Design review of the part built by this model. Coordinates are the model's own, in mm. Face numbers are marked on the shaded views. A direction names the side the tool comes from. Give positions to 0.01 mm unless a question says otherwise; leave off trailing zeros. Write each loop counter-clockwise with the first axis right and the second up, starting at its lowest first coordinate (ties: lowest second). Pieces come first, ordered by that corner, then holes.
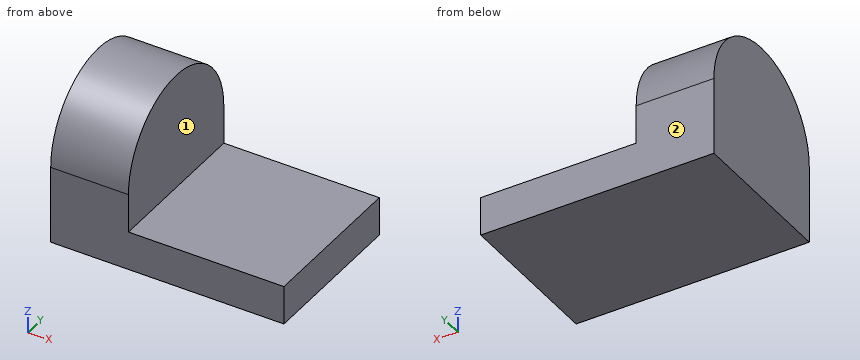
```python
from build123d import *

# Parameters (mm, degrees)
F0_W     = 152.4
F0_H     = 101.6
F1_DEPTH = 25.4
F2_W     = 101.6
F2_H     = 25.4
F3_DEPTH = 50.8


with BuildPart() as f1:
    # F0 (on Top) → F1 (new body)
    with BuildSketch(Plane.XY):
        with Locations((-76.2, 50.8)):
            Rectangle(F0_W, F0_H)
    extrude(amount=F1_DEPTH)

    # F2 (on face) → F3 (join)
    with BuildSketch(Plane(origin=(-152.4, 0, 0), x_dir=(0, -1, 0), z_dir=(-1, 0, 0))):
        with Locations((-50.8, 38.1)):
            Rectangle(F2_W, F2_H)
        with BuildLine():
            ThreePointArc((0, 50.8), (-50.8, 101.6), (-101.6, 50.8))
            Line((-101.6, 50.8), (0, 50.8))
        make_face()
    extrude(amount=-F3_DEPTH)


solid = f1.part
```
(1) Consider section C-C, the plane z = 36. Give the boundary of the cut face in (x, y).
Resolved:
outline: (-152.4, 0) - (-101.6, 0) - (-101.6, 101.6) - (-152.4, 101.6) - close
(2) To check wall thickness, follow L1, parallel to X at y = 15, z = 75.5; L2, parallel to Z at x = -117, y = 49.5; L3, parallel to Z at x = -33, y = 90. State the ranges of each line that lie inside material, in increasing order.
Resolved:
L1: x = -152.4 to -101.6
L2: z = 0 to 101.58
L3: z = 0 to 25.4
(3) Consider section A-A, the plane y = 50.8. Give the boundary of the cut face in (x, z).
Resolved:
outline: (-152.4, 0) - (0, 0) - (0, 25.4) - (-101.6, 25.4) - (-101.6, 101.6) - (-152.4, 101.6) - close
(4) Tool access review of the marked faces 1 and 2: name each direction out of +Z, -Z, +X, -X, +Y, -Y from which nothing blocks a thin tool from reaching the whole face with its end or side.
Resolved:
face 1: +Z, +X, +Y, -Y
face 2: +Z, -Z, +X, -X, +Y
(5) Clearance check with flat-ended pins moving along their axes: P1, Ø12, axis at x = -27.5, y = 20, coming from the +Z side; P2, Ø4, axis at x = -98.5, z = 54.5, coming from the +Y side (3 decimals); P3, Ø5, axis at y = 16.5, z = 62.5, coming from the +X side. State where each tip first meets the part, or that it passes through.
Resolved:
P1: stops at z = 25.4
P2: passes through
P3: stops at x = -101.6
(6) Consider section B-B, the plane x = -21. Give the boundary of the cut face in (y, z), then the cut area to 3 significant figures.
Resolved:
outline: (0, 0) - (101.6, 0) - (101.6, 25.4) - (0, 25.4) - close
area: 2,580 mm2
(7) Consider section D-D, the plane y = 82. Give the boundary of the cut face in (x, z).
Resolved:
outline: (-152.4, 0) - (0, 0) - (0, 25.4) - (-101.6, 25.4) - (-101.6, 90.89) - (-152.4, 90.89) - close
